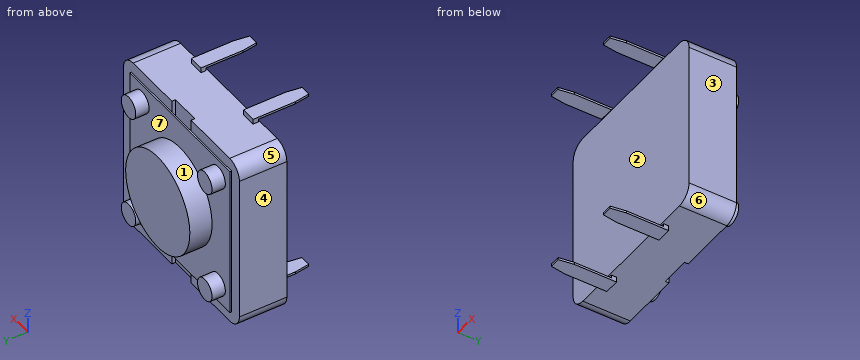
from build123d import *

# Parameters (mm, degrees)
SKETCH1_W           = 12
SKETCH1_H           = 12
BOSS_EXTRUDE1_DEPTH = 3.2
SKETCH2_R           = 0.75
BOSS_EXTRUDE2_DEPTH = 1
SKETCH3_W           = 10.4
SKETCH3_H           = 10.4
BOSS_EXTRUDE3_DEPTH = 0.1
SKETCH4_R           = 3.325
BOSS_EXTRUDE4_DEPTH = 1.5
FILLET1_R           = 1
SKETCH5_W           = 2
SKETCH5_H           = 12
CUT_EXTRUDE1_DEPTH  = 0.25
SKETCH6_W           = 1
SKETCH6_H           = 0.35
BOSS_EXTRUDE5_DEPTH = 0.35
SKETCH7_W           = 1
SKETCH7_H           = 0.15
BOSS_EXTRUDE6_DEPTH = 3.5
CUT_EXTRUDE4_DEPTH  = 18.876311141


with BuildPart() as part:
    # Sketch1 → Boss-Extrude1 (new body)
    with BuildSketch(Plane(origin=(0, 0, 0), x_dir=(1, 0, 0), z_dir=(0, 1, 0))):
        with Locations((6, 6)):
            Rectangle(SKETCH1_W, SKETCH1_H)
    extrude(amount=BOSS_EXTRUDE1_DEPTH)

    # Sketch2 → Boss-Extrude2 (add)
    with BuildSketch(Plane(origin=(0, 3.2, 0), x_dir=(1, 0, 0), z_dir=(0, 1, 0))):
        with Locations(Location((2.05, 9.95, 0), (0, 0, 90))):
            Circle(SKETCH2_R)
        with Locations(Location((9.95, 9.95, 0), (0, 0, 90))):
            Circle(SKETCH2_R)
        with Locations(Location((2.05, 2.05, 0), (0, 0, 90))):
            Circle(SKETCH2_R)
        with Locations(Location((9.95, 2.05, 0), (0, 0, 90))):
            Circle(SKETCH2_R)
    extrude(amount=BOSS_EXTRUDE2_DEPTH)

    # Sketch3 → Boss-Extrude3 (add)
    with BuildSketch(Plane(origin=(0, 3.2, 0), x_dir=(1, 0, 0), z_dir=(0, 1, 0))):
        with Locations((6, 6)):
            Rectangle(SKETCH3_W, SKETCH3_H)
    extrude(amount=BOSS_EXTRUDE3_DEPTH)

    # Sketch4 → Boss-Extrude4 (add)
    with BuildSketch(Plane(origin=(0, 3.3, 0), x_dir=(1, 0, 0), z_dir=(0, 1, 0))):
        with Locations(Location((6, 6, 0), (0, 0, 270))):
            Circle(SKETCH4_R)
    extrude(amount=BOSS_EXTRUDE4_DEPTH)

    # Fillet1
    fillet1_edges = [part.edges().sort_by_distance(p)[0] for p in [
        (0, 1.6, -12),
        (12, 1.6, -12),
        (12, 1.6, 0),
        (0, 1.6, 0),
    ]]
    fillet(fillet1_edges, radius=FILLET1_R)

    # Sketch5 → Cut-Extrude1 (cut)
    with BuildSketch(Plane(origin=(0, 3.2, 0), x_dir=(1, 0, 0), z_dir=(0, 1, 0))):
        with Locations((6, 6)):
            Rectangle(SKETCH5_W, SKETCH5_H)
    extrude(amount=-CUT_EXTRUDE1_DEPTH, mode=Mode.SUBTRACT)

    # Sketch6 → Boss-Extrude5 (add)
    with BuildSketch(Plane.XY):
        with Locations((3.3, 0.275)):
            Rectangle(SKETCH6_W, SKETCH6_H)
        with Locations((8.7, 0.275)):
            Rectangle(SKETCH6_W, SKETCH6_H)
    boss_extrude5 = extrude(amount=BOSS_EXTRUDE5_DEPTH)

    # Sketch7 → Boss-Extrude6 (add)
    with BuildSketch(Plane.XZ.offset(-0.1)):
        with Locations((3.3, 0.275)):
            Rectangle(SKETCH7_W, SKETCH7_H)
        with Locations((8.7, 0.275)):
            Rectangle(SKETCH7_W, SKETCH7_H)
    boss_extrude6 = extrude(amount=BOSS_EXTRUDE6_DEPTH)

    # Sketch8 → Cut-Extrude4 (cut, through all)
    with BuildSketch(Plane.XY.offset(0.35)):
        Polygon((2.95, -3.4), (2.8, -2.4), (2.8, -3.4), align=None)
        Polygon((3.8, -2.4), (3.65, -3.4), (3.8, -3.4), align=None)
        Polygon((8.2, -2.4), (8.35, -3.4), (8.2, -3.4), align=None)
        Polygon((9.2, -2.4), (9.05, -3.4), (9.2, -3.4), align=None)
    cut_extrude4 = extrude(amount=-CUT_EXTRUDE4_DEPTH, mode=Mode.SUBTRACT)

    # Mirror1: Boss-Extrude5, Boss-Extrude6, Cut-Extrude4 across plane
    add(boss_extrude5.mirror(Plane.XY.offset(-6)))
    add(boss_extrude6.mirror(Plane.XY.offset(-6)))
    add(cut_extrude4.mirror(Plane.XY.offset(-6)), mode=Mode.SUBTRACT)


solid = part.part
Work out the finished part from the listing and answer in its coordinate system (mm). Face numbers are marked on the shaded views. A direction names the side the tool comes from. Give positions to 0.01 mm unless a question says otherwise; leave off trailing zeros. Order: outer loops, then holes, each group sorted by start corner. A loop starts at its lowest first (then second) coordinate and runs counter-clockwise, first axis right, second up. Notation, with made-up numbers: (69.5, -7.75) - (73.5, -7.75) arc R33 ccw to (73.5, 25.25) - close; hole circle Ø3 at (40.25, -16.5). An arc over 180 degrees is marked (long way). Answer as CSV lines item,"result". Start each with the question number.
Q1. Find the intervals of material crossed by L1, parallel to Y at x = 5.25, z = -7.5; L2, parallel to X at y = 3, z = -2; L3, parallel to Y at x = 7.75, z = -10.75, in increasing order. Write a range as [from, to].
Q2. Given pin 1 Ø1.5 at (x, y) = (5.5, 2) entering from +Z; pin 2 Ø3 at (x, y) = (9.5, 2.5) entering from -Z; pin 3 Ø1.6 at (x, z) = (10, -2) entering from +Y, each flat-ended and moving along its own axis, determine where each tip first touches the part or whether it passes through.
Q3. The mould has two halves that part along Z. Classify the marked faces 4, 5, 6 and 7: +Z half, -Z half, draft (parallel to the pull), parting line (faces both ways), or undercut.
Q4. The part is cut by section A-A (x = 6). Write down the section's boundary in (y, z) (3 decimals).
Q5. The part is cut by section B-B (z = -9.5). Write down the section's boundary in (x, y), then the cut area to 3 significant figures.
Q6. The part is cut by section D-D (x = 9.95). Write down the section's boundary in (y, z), then the cut area to 3 significant figures.
Q7. The part is cut by section C-C (y = -1). Write down the section's boundary in (x, z).
Q8. For the marked faces 1, 2 and 3, determine the directions among +Z, -Z, +X, -X, +Y, -Y from which every point of the face is accessible in a straight line to the end or side of a thin tool.
Check result:
1,L1,"y = [0, 2.95], [3.2, 4.8]"
1,L2,"x = [0, 5], [7, 12]"
1,L3,"y = [0, 3.3]"
2,pin 1,"stops at z = 0"
2,pin 2,"stops at z = -12"
2,pin 3,"stops at y = 4.2"
3,face 4,"draft"
3,face 5,"+Z half"
3,face 6,"-Z half"
3,face 7,"undercut"
4,outline,"(0, -12) - (2.95, -12) - (2.95, 0) - (0, 0) - close; (3.2, -11.2) - (3.3, -11.2) - (3.3, -9.325) - (4.8, -9.325) - (4.8, -2.675) - (3.3, -2.675) - (3.3, -0.8) - (3.2, -0.8) - close"
5,outline,"(0, 0) - (12, 0) - (12, 3.2) - (11.2, 3.2) - (11.2, 3.3) - (10.55, 3.3) - (10.55, 4.2) - (9.35, 4.2) - (9.35, 3.3) - (2.65, 3.3) - (2.65, 4.2) - (1.45, 4.2) - (1.45, 3.3) - (0.8, 3.3) - (0.8, 3.2) - (0, 3.2) - close; hole (5, 2.95) - (7, 2.95) - (7, 3.2) - (5, 3.2) - close"
5,area,"41.1 mm²"
6,outline,"(0, -12) - (3.2, -12) - (3.2, -11.2) - (3.3, -11.2) - (3.3, -10.7) - (4.2, -10.7) - (4.2, -9.2) - (3.3, -9.2) - (3.3, -2.8) - (4.2, -2.8) - (4.2, -1.3) - (3.3, -1.3) - (3.3, -0.8) - (3.2, -0.8) - (3.2, 0) - (0, 0) - close"
6,area,"42.1 mm²"
7,outline,"(2.8, -12.35) - (3.8, -12.35) - (3.8, -12.2) - (2.8, -12.2) - close; (2.8, 0.2) - (3.8, 0.2) - (3.8, 0.35) - (2.8, 0.35) - close; (8.2, -12.35) - (9.2, -12.35) - (9.2, -12.2) - (8.2, -12.2) - close; (8.2, 0.2) - (9.2, 0.2) - (9.2, 0.35) - (8.2, 0.35) - close"
8,face 1,"+Y"
8,face 2,"+X, -X, -Y"
8,face 3,"+Z, -Z, +X, +Y, -Y"
